The model under review builds one solid part; all positions refer to its coordinate system, in mm. A direction names the side the tool comes from. Round coordinates to 2 decimals unless told otherwise and drop trailing zeros. Order: outer loops, then holes, each group sorted by start corner. A loop starts at its lowest first (then second) coordinate and runs counter-clockwise, first axis right, second up. Notation, with made-up numbers: M 7.25,15 L 60.25,15 A12 ccw 60.25,32 Z; hole C 7,19.25 d6. An arc over 180 degrees is marked long. One line per item, written item: value. Start each with the question number.
from build123d import *

# Parameters (mm, degrees)
CUT_EXTRUDE3_DEPTH      = 4.5
CUT_EXTRUDE3_DEPTH_BACK = 4.5


with BuildPart() as part:
    # Sketch1 → Revolve1 (revolve)
    with BuildSketch(Plane.XY):
        Polygon((10.63699913, 3), (6.13699913, 3.5), (6.13699913, 2.5), (5.38699913, 2.5), (1.38699913, 3.5), (1.38699913, 2.5), (-4.354665221, 2.5), (-4.354665221, 2), (10.63699913, 2), align=None)
    revolve(axis=Axis((0, 0, 0), (1, 0, 0)))

    # Sketch2 → Cut-Extrude3 (cut, two sides)
    with BuildSketch(Plane.XY) as cut_extrude3_sk:
        Polygon((-1.854665221, 2.5), (-4.354665221, 2.5), (-4.354665221, 0), align=None)
        Polygon((-4.354665221, -2.5), (-4.354665221, 0), (-1.854665221, -2.5), align=None)
    extrude(amount=CUT_EXTRUDE3_DEPTH, mode=Mode.SUBTRACT)
    extrude(cut_extrude3_sk.sketch, amount=-CUT_EXTRUDE3_DEPTH_BACK, mode=Mode.SUBTRACT)


solid = part.part
Item 1: Clearance check with flat-ended pins moving along their axes: P1, Ø2, axis at y = -0.5, z = 0.5, coming from the -X side; P2, Ø4, axis at x = 2, z = 2, coming from the +Y side; P3, Ø1, axis at x = 5, y = 2, coming from the +Z side. State where each tip first meets the part, or that it passes through.
Item 2: Consider section B-B, the plane x = -0.25. Give the boundary of the cut face in (y, z), then the cut area to 3 significant figures.
Item 3: The part is to be moulded in two halves that separate along Z. For faces 4 (the flat face through (10.637, -1, -2)), 5 (the conical face through (8.855, -2.538, -1.946)), 6 (the cylindrical face through (3, 0, -2)), say which applies: pulls with the +Z half, pulls with the -Z half, needs draft (parallel to the pull), parting line crosses it, or undercut.
Item 4: Consider section C-C, the plane x = 3.5. Give the boundary of the cut face in (y, z), then the cut area to 3 significant figures.
Item 5: Machinability: for faces 1 (the flat face through (-2.277, -2.077, 0.567)), 2 (the flat face through (6.137, 2, -2)), 3 (the cylindrical face through (-0.9, -2.5, 0.1)), which of the approach directions +Z, -Z, +X, -X, +Y, -Y give a long, thin tool a straight path to every point of the face, cutting with its end or side? Answer none if there is none.
Item 6: Wall thickness on L1, parallel to Z at x = -1.5, y = 0; L2, parallel to Z at x = 2.25, y = 1.5; L3, parallel to Y at x = -1.25, z = 1.25: over which ranges is each line inside the solid? List them lowest first.
Item 7: Consider section A-A, the plane z = 0. Give the boundary of the cut face in (x, y), then the cut area to 3 significant figures.
Computed:
1. P1: passes through
1. P2: stops at y = 3.5
1. P3: stops at z = 2.15
2. outline: C 0,0 d5; hole C 0,0 d4
2. area: 7.07 mm^2
3. face 4: needs draft
3. face 5: parting line crosses it
3. face 6: undercut
4. outline: C 0,0 d5.94; hole C 0,0 d4
4. area: 15.2 mm^2
5. face 1: +Z, -Z, -X, -Y
5. face 2: none
5. face 3: -X
6. L1: z = -2.5 to -2, 2 to 2.5
6. L2: z = -2.92 to -1.32, 1.32 to 2.92
6. L3: y = -2.17 to -1.56, 1.56 to 2.17
7. outline: M -2.35,-2 L -1.85,-2.5 L 1.39,-2.5 L 1.39,-3.5 L 5.39,-2.5 L 6.14,-2.5 L 6.14,-3.5 L 10.64,-3 L 10.64,-2 Z; M -2.35,2 L 10.64,2 L 10.64,3 L 6.14,3.5 L 6.14,2.5 L 5.39,2.5 L 1.39,3.5 L 1.39,2.5 L -1.85,2.5 Z
7. area: 23.5 mm^2
